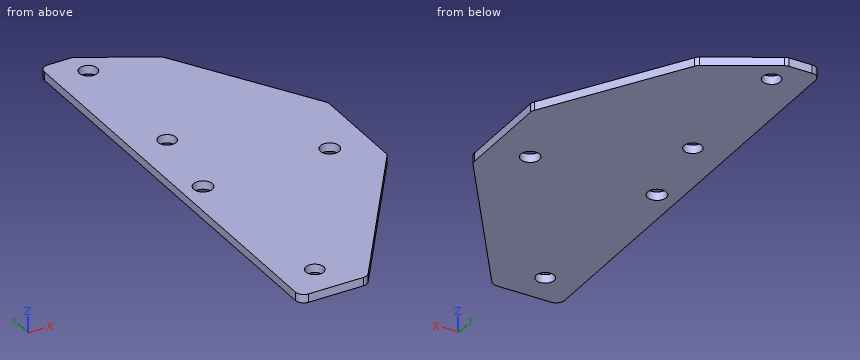
Autodesk Inventor part; units mm, degrees
ref_plane "YZ Plane" through (0, 0, 0) normal (1, 0, 0) x (0, 1, 0)
ref_plane "XZ Plane" through (0, 0, 0) normal (0, 1, 0) x (-1, 0, 0)
ref_plane "XY Plane" through (0, 0, 0) normal (0, 0, 1) x (1, 0, 0)
sketch "Sketch1" plane through (0, 0, 0) normal (0, 0, 1) x (1, 0, 0)
  line L0 (69.85, 0) -> (69.85, 38.1)
  line L1 (69.85, 38.1) -> (29.1042, 104.775)
  line L2 (0, 104.775) -> (0, 0)
  line L3 (0, -63.5) -> (0, 0)
  line L4 (0, 104.775) -> (29.1042, 104.775)
  line L5 (0, -63.5) -> (25.4, -63.5)
  line L6 (25.4, -63.5) -> (69.85, 0)
  dimension "d1" = 38.1
  dimension "d24" = 63.5
  dimension "d25" = 69.85
  dimension "d26" = 69.85
  dimension "d36" = 104.775
  dimension "d38" = 121.43
  dimension "d45" = 25.4
extrude "Extrusion1" add sketch "Sketch1" along normal blind 3.175
sketch "Sketch2" plane through (0, 0, 3.175) normal (0, 0, 1) x (1, 0, 0)
  line L0 (0, 0) -> (69.85, 0)
  line L1 (69.85, 0) -> (69.85, 38.1)
  line L2 (0, 104.775) -> (0, -63.5)
  circle A0 centre (7.874, 12.7) radius 3.556
  circle A1 centre (55.626, 12.7) radius 3.556
  point P0 (0, 152.4)
  dimension "d5" = 7.112
  dimension "d6" = 7.112
  dimension "d7" = 12.7
  dimension "d8" = 12.7
  dimension "d9" = 14.224
  dimension "d11" = 7.874
extrude "Extrusion2" cut sketch "Sketch2" against normal blind 25.4
sketch "Sketch3" plane through (0, 0, 3.175) normal (0, 0, 1) x (1, 0, 0)
  line L0 (0, 104.775) -> (0, -63.5)
  line L1 (0, 0) -> (69.85, 0)
  circle A0 centre (12.7, 94.9198) radius 3.3782
  circle A1 centre (12.7, 44.1198) radius 3.3782
  point P0 (0, 141.1158)
  dimension "d15" = 6.7564
  dimension "d16" = 6.7564
  dimension "d17" = 12.7
  dimension "d18" = 12.7
  dimension "d19" = 44.1198
  dimension "d20" = 50.8
extrude "Extrusion3" cut sketch "Sketch3" against normal blind 25.4
fillet "Fillet2" radius 3.175 2 edges at (69.85, 0, 1.5875) (69.85, 38.1, 1.5875)
fillet "Fillet3" radius 3.175 1 edges at (0, -63.5, 1.5875)
sketch "Sketch4" plane through (0, 0, 3.175) normal (0, 0, 1) x (1, 0, 0)
  line L0 (0, 104.775) -> (0, -60.325)
  circle A0 centre (12.7, 44.1198) radius 3.3782
  circle A1 centre (12.7, -51.1302) radius 3.3782
  point P0 (0, 141.1158)
  point P1 (0, 0)
  dimension "d28" = 6.7564
  dimension "d29" = 95.25
  dimension "d30" = 12.7
extrude "Extrusion4" cut sketch "Sketch4" against normal blind 25.4 contours A1
sketch "Sketch5" plane through (0, 0, 3.175) normal (0, 0, 1) x (1, 0, 0)
  circle A0 centre (12.7, 44.1198) radius 3.3782
  circle A1 centre (12.7, 94.9198) radius 3.3782
  point P0 (0, 0)
extrude "Extrusion5" cut sketch "Sketch5" against normal blind 25.4
fillet "Fillet4" radius 3.175 2 edges at (29.1042, 104.775, 1.5875) (0, 104.775, 1.5875)
sketch "Sketch6" plane through (0, 0, 3.175) normal (0, 0, 1) x (1, 0, 0)
  line L0 (0, 101.6) -> (0, -60.325)
  line L1 (69.3842, 38.8623) -> (30.0327, 103.2556)
  arc A0 (30.0327, 103.2556) -> (27.3235, 104.775) centre (27.3235, 101.6) ccw
  line L2 (27.3235, 104.775) -> (3.175, 104.775)
  line L3 (12.7, 104.775) -> (38.0473, 90.1407)
  point P0 (0, 0)
  dimension "d40" = 30
  dimension "d41" = 12.7
extrude "Extrusion6" cut sketch "Sketch6" against normal blind 25.4
fillet "Fillet5" radius 3.175 2 edges at (12.7, 104.775, 1.5875) (38.0473, 90.1407, 1.5875)
fillet "Fillet6" radius 3.175 1 edges at (25.4, -63.5, 1.5875)
properties part number "Ninja left cylinder support bracket"
Model file for the job. Use its own axes, mm. Give positions to 0.01 mm unless a question says otherwise; leave off trailing zeros. Order: outer loops, then holes, each group sorted by start corner. A loop starts at its lowest first (then second) coordinate and runs counter-clockwise, first axis right, second up.
1) Wall check: probe 1 along Y at (x, z) = (13, 2.6); probe 2 along Y at (x, z) = (6, 1) (3 decimals); probe 3 along X at (y, z) = (93, 1.9). Give the ranges that are in metal, low to high.
2) Saw through at C-C, the plane y = -40. Write the cut outline in (x, z) (3 decimals), then the cut area to 3 significant figures.
3) Saw through at B-B, the plane z = 1.6. Write the cut outline in (x, y) (3 decimals).
4) Saw through at D-D, the plane x = 41.5. Write the cut outline in (y, z) (3 decimals).
5) Pin check, flat tip, straight feed: pin 1 (6 mm diameter, centred on x = 12.7, y = 44.12, fed in from -Z). Stop position of the tip, or through.
6) Saw through at A-A, the plane y = 12.7. Write the cut outline in (x, z) (3 decimals), then the cut area to 3 significant figures.
Computed:
1. probe 1: y = -63.5 to -54.5, -47.77 to 40.75, 47.48 to 91.55, 98.28 to 104.56
1. probe 2: y = -63.5 to 9.678, 15.722 to 104.775
1. probe 3: x = 0 to 9.92, 15.48 to 33.09
2. outline: (0, 0) - (41.85, 0) - (41.85, 3.175) - (0, 3.175) - close
2. area: 133 mm2
3. outline: (0, -60.325) arc R3.175 ccw to (3.175, -63.5) - (23.747, -63.5) arc R3.175 ccw to (26.348, -62.146) - (69.276, -0.82) arc R3.175 ccw to (69.85, 1.001) - (69.85, 37.207) arc R3.175 ccw to (69.384, 38.862) - (38.469, 89.451) arc R3.175 ccw to (37.347, 90.545) - (13.437, 104.35) arc R3.175 ccw to (11.849, 104.775) - (3.175, 104.775) arc R3.175 ccw to (0, 101.6) - close; hole circle Ø7.112 at (7.874, 12.7); hole circle Ø6.756 at (12.7, -51.13); hole circle Ø6.756 at (12.7, 44.12); hole circle Ø6.756 at (12.7, 94.92); hole circle Ø7.112 at (55.626, 12.7)
4. outline: (-40.5, 0) - (84.491, 0) - (84.491, 3.175) - (-40.5, 3.175) - close
5. pin 1: passes through
6. outline: (0, 0) - (4.318, 0) - (4.318, 3.175) - (0, 3.175) - close; (11.43, 0) - (52.07, 0) - (52.07, 3.175) - (11.43, 3.175) - close; (59.182, 0) - (69.85, 0) - (69.85, 3.175) - (59.182, 3.175) - close
6. area: 177 mm2
